Model file for the job. Use its own axes, mm. A direction names the side the tool comes from. Give positions to 0.01 mm unless a question says otherwise; leave off trailing zeros. Loops run counter-clockwise (first coordinate to the right, second up) from the corner with the lowest first, then second, coordinate; pieces in that order, holes last. Notation, with made-up numbers: M 36,69 L 58,69 A8 ccw 58,76 Z; hole C 18,-7 d10. An arc over 180 degrees is marked long. Answer in a Markdown table with one row per item.
```python
from build123d import *

# Parameters (mm, degrees)
SKETCH1_R           = 4.25
BOSS_EXTRUDE1_DEPTH = 5.3
SKETCH2_R           = 2.5
BOSS_EXTRUDE2_DEPTH = 3
SHELL2_T            = -0.7
FILLET1_R           = 1
SKETCH3_R           = 0.4
BOSS_EXTRUDE4_DEPTH = 0.6


with BuildPart() as part:
    # Sketch1 → Boss-Extrude1 (new body)
    with BuildSketch(Plane(origin=(0, 0, 0), x_dir=(1, 0, 0), z_dir=(0, 1, 0))):
        with Locations(Location((0, 0, 0), (0, 0, 270))):
            Circle(SKETCH1_R)
    extrude(amount=BOSS_EXTRUDE1_DEPTH)

    # Sketch2 → Boss-Extrude2 (add)
    with BuildSketch(Plane.XZ):
        with Locations(Location((0, 0, 0), (0, 0, 90))):
            Circle(SKETCH2_R)
    extrude(amount=BOSS_EXTRUDE2_DEPTH)

    # Shell2
    shell2_openings = [part.faces().sort_by_distance(p)[0] for p in [
        (0, -3, 0),
    ]]
    offset(amount=SHELL2_T, openings=shell2_openings, kind=Kind.INTERSECTION)

    # Fillet1
    fillet1_edges = [part.edges().sort_by_distance(p)[0] for p in [
        (0, 5.3, -4.25),
    ]]
    fillet(fillet1_edges, radius=FILLET1_R)

    # Sketch3 → Boss-Extrude4 (add)
    with BuildSketch(Plane(origin=(0, 5.3, 0), x_dir=(1, 0, 0), z_dir=(0, 1, 0))):
        with Locations(Location((0, -2.25, 0), (0, 0, 270))):
            Circle(SKETCH3_R)
        with BuildLine():
            ThreePointArc((0.966334519, -0.786985884), (0, -0.4), (-0.966334519, -0.786985884))
            ThreePointArc((-0.966334519, -0.786985884), (-0.979671546, -1.352514066), (-0.414143365, -1.365851093))
            ThreePointArc((-0.414143365, -1.365851093), (0, -1.2), (0.414143365, -1.365851093))
            ThreePointArc((0.414143365, -1.365851093), (0.979671546, -1.352514066), (0.966334519, -0.786985884))
        make_face()
        with BuildLine():
            ThreePointArc((1.545056478, 0.405803093), (0, 1.2), (-1.545056478, 0.405803093))
            ThreePointArc((-1.545056478, 0.405803093), (-1.452582081, -0.152272606), (-0.894506382, -0.059798209))
            ThreePointArc((-0.894506382, -0.059798209), (0, 0.4), (0.894506382, -0.059798209))
            ThreePointArc((0.894506382, -0.059798209), (1.452582081, -0.152272606), (1.545056478, 0.405803093))
        make_face()
        with BuildLine():
            ThreePointArc((2.32, 1.49), (0, 2.65), (-2.32, 1.49))
            ThreePointArc((-2.32, 1.49), (-2.24, 0.93), (-1.68, 1.01))
            ThreePointArc((-1.68, 1.01), (0, 1.85), (1.68, 1.01))
            ThreePointArc((1.68, 1.01), (2.24, 0.93), (2.32, 1.49))
        make_face()
    extrude(amount=BOSS_EXTRUDE4_DEPTH)


solid = part.part
```
(1) Which spindle directions (+Z, -Z, +X, -X, +Y, -Y) get a long thin tool onto all of the face, cutting with end or side? Do faces 4 (the cylindrical face through (2.44, -1.48, -0.54)), 5 (the cylindrical face through (0.04, 5.6, -2.65)), 6 (the flat face through (1, 0.7, -2)), 7 (the cylindrical face through (-0.03, 5.6, -1.85)). Say none if no direction does.
Established:
| item | result |
|---|---|
| face 4 | -Y |
| face 5 | -Z, +Y |
| face 6 | none |
| face 7 | +Y |
(2) Wall check: L1, parallel to Y at x = -2, z = 0.75; L2, parallel to Y at x = 2.75, z = -1.25; L3, parallel to X at y = -0.7, z = 0. Give the ranges that are in metal, low to high.
Established:
| item | result |
|---|---|
| L1 | y = -3 to 0.7, 4.6 to 5.3 |
| L2 | y = 0 to 0.7, 4.6 to 5.3 |
| L3 | x = -2.5 to -1.8, 1.8 to 2.5 |
(3) Saw through at C-C, the plane y = 1.5. Give the cut face in (x, z), and give its area (3 significant figures).
Established:
| item | result |
|---|---|
| outline | C 0,0 d8.5; hole C 0,0 d7.1 |
| area | 17.2 mm2 |
(4) Flat gauge pins, fed straight in: P1, Ø5, axis at x = 3, y = 0.5, coming from the +Z side; P2, Ø3, axis at y = 2.5, z = 3.5, coming from the -X side; P3, Ø1.5, axis at x = 2, y = 3, coming from the +Z side. Where does each tip first touch, or does it go through?
Established:
| item | result |
|---|---|
| P1 | stops at z = 4.22 |
| P2 | stops at x = -3.75 |
| P3 | stops at z = 4.06 |
(5) Saw through at B-B, the plane y = -1. Give the cut face in (x, z), and give its area (3 significant figures).
Established:
| item | result |
|---|---|
| outline | C 0,0 d5; hole C 0,0 d3.6 |
| area | 9.46 mm2 |
(6) Mould opens along X. For faces 1 (the cylindrical face through (4.214, 2.12, -0.553)), 2 (the flat face through (-2, 0, 2)), 3 (the cylindrical face through (0.689, -1.124, 1.663)) say: pulls with the +X half, pulls with the -X half, needs draft (parallel to the pull), parting line crosses it, or undercut.
Established:
| item | result |
|---|---|
| face 1 | parting line crosses it |
| face 2 | needs draft |
| face 3 | undercut |
